Source: CAD feature listing. Evaluate the final solid. Frame: model axes, mm. A direction names the side the tool comes from. Coordinates: 2 decimals unless noted, no trailing zeros. Order: outer loops, then holes, each group sorted by start corner. A loop starts at its lowest first (then second) coordinate and runs counter-clockwise, first axis right, second up. Notation, with made-up numbers: (34.5, -11) -> (76.5, -11) arc R13 ccw to (76.5, -2) -> close; hole circle Ø3 at (50.25, 37.25). An arc over 180 degrees is marked (long way). Write each question's results on one line, items separated by ' | '. Start each with the question number.
from build123d import *

# Parameters (mm, degrees)
F0_W     = 250
F0_H     = 150
F2_DEPTH = 15
F1_R     = 20.5
F3_DEPTH = 10
F4_DEPTH = 10
F5_DEPTH = 10
F6_DEPTH = 10
F7_DEPTH = 10
F8_DEPTH = 10


with BuildPart() as f2:
    # F0 (on Front) → F2 (new body)
    with BuildSketch(Plane.XZ):
        with Locations((-0.132803, 4.857429)):
            Rectangle(F0_W, F0_H)
    extrude(amount=F2_DEPTH)

    # F1 (on face) → F3 (cut)
    with BuildSketch(Plane.XZ):
        with Locations((57.814665, 52.574778)):
            Circle(F1_R)
    extrude(amount=F3_DEPTH, mode=Mode.SUBTRACT)

    # F1 (on face) → F4 (cut)
    with BuildSketch(Plane.XZ):
        with Locations((102.183415, 19.949049)):
            Circle(F1_R)
    extrude(amount=F4_DEPTH, mode=Mode.SUBTRACT)

    # F1 (on face) → F5 (cut)
    with BuildSketch(Plane.XZ):
        with Locations((102.183415, 19.949049)):
            Circle(F1_R)
    extrude(amount=-F5_DEPTH, mode=Mode.SUBTRACT)

    # F1 (on face) → F6 (cut)
    with BuildSketch(Plane.XZ):
        with Locations((88.780629, -33.229924)):
            Circle(F1_R)
    extrude(amount=F6_DEPTH, mode=Mode.SUBTRACT)

    # F1 (on face) → F7 (cut)
    with BuildSketch(Plane.XZ):
        with Locations((30.196567, -33.758188)):
            Circle(F1_R)
    extrude(amount=F7_DEPTH, mode=Mode.SUBTRACT)

    # F1 (on face) → F8 (cut)
    with BuildSketch(Plane.XZ):
        with Locations((15.077671, 17.431745)):
            Circle(F1_R)
    extrude(amount=F8_DEPTH, mode=Mode.SUBTRACT)


solid = f2.part
(1) Draft query along Z for faces 3 (the flat face through (58, -10, 53)), 4 (the cylindrical face through (42.705, -4.93, 66.43)), 5 (the flat face through (124.867, -7, 4)), 6 (the flat face through (-2, -7, -70.143)). Return one class per face: released by +Z, released by -Z, zero draft, split by the parting line, or undercut.
(2) Section C-C on x = 64.5. Return the cut outline in (y, z), then the cut area to 3 significant figures.
(3) First-contact query: P1, Ø12.5, axis at x = 60.5, z = 54.5, coming from the +Y side. Flat tip, straight axial feed; report the tip coordinate or a pass-through.
(4) Section B-B on z = 12. Return the cut outline in (x, y), then the cut area to 3 significant figures.
(5) Section D-D on z = 58. Return the cut outline in (x, y), then the cut area to 3 significant figures.
(6) Line query: L1, parallel to X at y = -8.5, z = -30; L2, parallel to X at y = -0.75, z = -18; L3, parallel to Z at x = 98, y = -4.5. Output: solid intervals per line, ascending.
(7) Section A-A on y = -6. Return the cut outline in (x, z), then the cut area to 3 significant figures.
(8) Reachability of faces 1 (the flat face through (102, -10, 20)), 2 (the flat face through (-2, -15, 6)) from +Z, -Z, +X, -X, +Y, -Y: full face, straight path, thin tool, end or side. Return the list, or none.
Results list:
1) face 3: undercut | face 4: undercut | face 5: zero draft | face 6: released by -Z
2) outline: (-15, -70.14) -> (0, -70.14) -> (0, 33.2) -> (-10, 33.2) -> (-10, 71.95) -> (0, 71.95) -> (0, 79.86) -> (-15, 79.86) -> close | area: 1,860 mm²
3) P1: stops at y = -10
4) outline: (-125.13, -15) -> (124.87, -15) -> (124.87, 0) -> (121.08, 0) -> (121.08, -10) -> (83.29, -10) -> (83.29, 0) -> (34.84, 0) -> (34.84, -10) -> (-4.69, -10) -> (-4.69, 0) -> (-125.13, 0) -> close | area: 2,980 mm²
5) outline: (-125.13, -15) -> (124.87, -15) -> (124.87, 0) -> (77.58, 0) -> (77.58, -10) -> (38.05, -10) -> (38.05, 0) -> (-125.13, 0) -> close | area: 3,350 mm²
6) L1: x = -125.13 to 10.04, 50.35 to 68.54, 109.02 to 124.87 | L2: x = -125.13 to 17.08, 43.31 to 75.06, 102.5 to 124.87 | L3: z = -70.14 to -51.54, -14.92 to -0.12, 40.02 to 79.86
7) outline: (-125.13, -70.14) -> (124.87, -70.14) -> (124.87, 79.86) -> (-125.13, 79.86) -> close; hole circle Ø41 at (15.08, 17.43); hole circle Ø41 at (30.2, -33.76); hole circle Ø41 at (57.81, 52.57); hole circle Ø41 at (88.78, -33.23); hole circle Ø41 at (102.18, 19.95) | area: 30,900 mm²
8) face 1: +Y | face 2: +Z, -Z, +X, -X, -Y
